from build123d import *

# Parameters (mm, degrees)
BOSS_EXTRUDE1_DEPTH = 1.000000032
SKETCH2_W           = 4.49999989
SKETCH2_H           = 5.735208424
SKETCH2_W_2         = 3
SKETCH2_H_2         = 2
BOSS_EXTRUDE2_DEPTH = 1
SKETCH3_W           = 4.300000036
SKETCH3_H           = 8.29999991
BOSS_EXTRUDE3_DEPTH = 3.000000096


with BuildPart() as part:
    # Sketch1 → Boss-Extrude1 (new body)
    with BuildSketch(Plane(origin=(0, 0, 0), x_dir=(1, 0, 0), z_dir=(0, 1, 0))):
        Polygon((-3.499999985, 9.50000005), (-0.499999889, 12.500000146), (0.499999889, 12.500000146), (3.499999985, 9.50000005), (4.999999906, 9.50000005), (20.000000132, 9.50000005), (20.000000132, -9.50000005), (4.999999906, -9.50000005), (3.499999985, -9.50000005), (0.499999889, -12.500000146), (-0.499999889, -12.500000146), (-3.499999985, -9.50000005), (-4.999999906, -9.50000005), (-4.999999906, 9.50000005), align=None)
    extrude(amount=-BOSS_EXTRUDE1_DEPTH)

    # Sketch2 → Boss-Extrude2 (add)
    with BuildSketch(Plane(origin=(0, 0, 0), x_dir=(1, 0, 0), z_dir=(0, 1, 0))):
        Rectangle(SKETCH2_W, SKETCH2_H)
        with Locations((-1.5875, 5.842)):
            Rectangle(SKETCH2_W_2, SKETCH2_H_2)
    extrude(amount=BOSS_EXTRUDE2_DEPTH)

    # Sketch3 → Boss-Extrude3 (add)
    with BuildSketch(Plane(origin=(0, 0, 0), x_dir=(1, 0, 0), z_dir=(0, 1, 0))):
        with Locations((16.580000114, 0)):
            Rectangle(SKETCH3_W, SKETCH3_H)
    extrude(amount=BOSS_EXTRUDE3_DEPTH)


solid = part.part
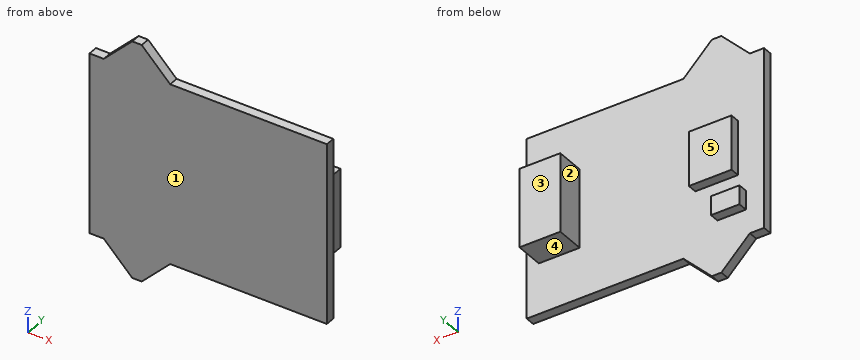
Build history of the part. All positions in model axes, mm. Face numbers are marked on the shaded views. A direction names the side the tool comes from. Coordinates: 2 decimals unless noted, no trailing zeros. Order: outer loops, then holes, each group sorted by start corner. A loop starts at its lowest first (then second) coordinate and runs counter-clockwise, first axis right, second up. Notation, with made-up numbers: (-30, 39) - (9, 39) arc R20 cw to (9, 70) - close; hole circle Ø5 at (1.25, 41.5). An arc over 180 degrees is marked (long way). Put each result on its own line as item: value.
1. Saw through at A-A (y = 0.5). Write the cut outline in (x, z).
Answer sheet:
outline: (-3.09, -6.84) - (-0.09, -6.84) - (-0.09, -4.84) - (-3.09, -4.84) - close; (-2.25, -2.87) - (2.25, -2.87) - (2.25, 2.87) - (-2.25, 2.87) - close; (14.43, -4.15) - (18.73, -4.15) - (18.73, 4.15) - (14.43, 4.15) - close
2. Saw through at C-C (x = -1.25). Write the cut outline in (y, z), and give its area (3 significant figures).
Answer sheet:
outline: (-1, -11.75) - (0, -11.75) - (0, -6.84) - (1, -6.84) - (1, -4.84) - (0, -4.84) - (0, -2.87) - (1, -2.87) - (1, 2.87) - (0, 2.87) - (0, 11.75) - (-1, 11.75) - close
area: 31.2 mm^2
3. Pull direction X, two halves, no side cores. Call the marked faces 1 and 2: pulls with the +X half, pulls with the -X half, needs draft (parallel to the pull), parting line crosses it, or undercut.
Answer sheet:
face 1: needs draft
face 2: undercut
4. Drop flat-ended pins along their axis: P1, Ø0.8, axis at y = 0.5, z = 1, coming from the +X side; P2, Ø0.8, axis at x = 9.5, y = -0.5, coming from the -Z side; P3, Ø0.5, axis at y = 0.5, z = -5.5, coming from the +X side. Give the stop position or say it passes through.
Answer sheet:
P1: stops at x = 18.73
P2: stops at z = -9.5
P3: stops at x = -0.09
5. Saw through at B-B (z = 1.25). Write the cut outline in (x, y), and give its area (3 significant figures).
Answer sheet:
outline: (-5, -1) - (20, -1) - (20, 0) - (18.73, 0) - (18.73, 3) - (14.43, 3) - (14.43, 0) - (2.25, 0) - (2.25, 1) - (-2.25, 1) - (-2.25, 0) - (-5, 0) - close
area: 42.4 mm^2
6. Probe line 1 along Y through (x, z) = (9.75, 1.25); line 2 along X through (y, z) = (1.6, -0.25); line 3 along Y through (x, z) = (-0.5, -1.5). List the from-to ranges inside material, lowest first. Write a range as [from, to].
Answer sheet:
line 1: y = [-1, 0]
line 2: x = [14.43, 18.73]
line 3: y = [-1, 1]
7. Saw through at D-D (x = 15.5). Write the cut outline in (y, z).
Answer sheet:
outline: (-1, -9.5) - (0, -9.5) - (0, -4.15) - (3, -4.15) - (3, 4.15) - (0, 4.15) - (0, 9.5) - (-1, 9.5) - close
8. Tool access for the marked faces 3, 4 and 5: list every direction of +Z, -Z, +X, -X, +Y, -Y with a clear straight run to the whole face (end or side of a thin tool).
Answer sheet:
face 3: +Z, -Z, +X, -X, +Y
face 4: -Z, +X, -X, +Y
face 5: +Z, -Z, -X, +Y
